The model under review builds one solid part; all positions refer to its coordinate system, in mm. A direction names the side the tool comes from. Coordinates: 2 decimals unless noted, no trailing zeros.
1) For line 1 (X direction, y = 10.75, z = -116); line 2 (Z direction, x = 81, y = 1); line 3 (Z direction, x = 41, y = 1), list the stretches that pass through material, from the lowest coordinate up.
2) For P1, Ø12.5, axis at x = -25.4, z = 50.8, coming from the +Y side; P2, Ø6, axis at x = -48.26, z = 31.75, coming from the -Y side; P3, Ø6, axis at x = 85, y = 6, coming from the +Z side, all flat-tipped, find the tip position at first contact; note any pin that passes through.
3) Machinability: for faces 5 (the cylindrical face through (0.151, 7.982, 105.794)), 6 (the cylindrical face through (-51.302, 3.187, 33.332)), 7 (the flat face through (124, 0, 30)), which of the approach directions +Z, -Z, +X, -X, +Y, -Y give a long, thin tool a straight path to every point of the face, cutting with its end or side? Answer none if there is none.
4) Mouldability with a two-part tool opening along Z and no side actions: class faces 1 (the cylindrical face through (60.55, 3.19, -0.45)), 2 (the cylindrical face through (136.38, 8.92, -30.28)), 3 (the flat face through (-2, 11.112, 2)), 4 (the cylindrical face through (-51.302, 3.187, -30.168)) as released by +Z, released by -Z, zero draft, split by the parting line, or undercut.
from build123d import *

# Parameters (mm, degrees)
SKETCH2_R          = 6.858
CUT_EXTRUDE1_DEPTH = 198.877910986
SKETCH3_R          = 25.4
SKETCH3_R_2        = 31.75
CUT_EXTRUDE3_DEPTH = 198.877910986
CUT_EXTRUDE4_START = -4.826
SKETCH4_R          = 3.429
CUT_EXTRUDE4_DEPTH = 6.35
SKETCH6_R          = 3.429
CUT_EXTRUDE6_DEPTH = 6.35


with BuildPart() as part:
    # Sketch1 → Revolve2 (revolve)
    with BuildSketch(Plane.XY, mode=Mode.PRIVATE) as revolve2_sk:
        with BuildLine():
            ThreePointArc((139.7, 6.7945), (136.8425, 3.937), (139.7, 1.0795))
            Line((139.7, 1.0795), (139.7, 0))
            Line((139.7, 0), (127, 0))
            Line((127, 0), (127, 2.54))
            Line((127, 2.54), (120.65, 2.54))
            Line((120.65, 2.54), (120.65, 0))
            Line((120.65, 0), (0, 0))
            Line((0, 0), (0, 11.1125))
            Line((0, 11.1125), (130.81, 11.1125))
            Line((130.81, 11.1125), (130.81, 9.8425))
            Line((130.81, 9.8425), (137.16, 9.8425))
            Line((137.16, 9.8425), (137.16, 11.1125))
            Line((137.16, 11.1125), (139.7, 11.1125))
            Line((139.7, 11.1125), (139.7, 6.7945))
        make_face()
    revolve(revolve2_sk.sketch.rotate(Axis((0, 28.20697446, 0), (0, -1, 0)), 90), axis=Axis((0, 28.20697446, 0), (0, -1, 0)))

    # Sketch2 → Cut-Extrude1 (cut, through all)
    with BuildSketch(Plane(origin=(0, 11.1125, 0), x_dir=(1, 0, 0), z_dir=(0, 1, 0))):
        with Locations(Location((-25.4, -50.8, 0), (0, 0, 270))):
            Circle(SKETCH2_R)
        with Locations(Location((25.4, -50.8, 0), (0, 0, 270))):
            Circle(SKETCH2_R)
    extrude(amount=-CUT_EXTRUDE1_DEPTH, mode=Mode.SUBTRACT)

    # Sketch3 → Cut-Extrude3 (cut, through all)
    with BuildSketch(Plane(origin=(0, 11.1125, 0), x_dir=(1, 0, 0), z_dir=(0, 1, 0))):
        with Locations(Location((0, 50.8, 0), (0, 0, 270))):
            Circle(SKETCH3_R)
        with Locations(Location((-82.55, 0, 0), (0, 0, 270))):
            Circle(SKETCH3_R_2)
    extrude(amount=-CUT_EXTRUDE3_DEPTH, mode=Mode.SUBTRACT)

    # Sketch4 → Cut-Extrude4 (cut)
    with BuildSketch(Plane(origin=(0, 11.1125, 0), x_dir=(1, 0, 0), z_dir=(0, 1, 0)).offset(CUT_EXTRUDE4_START)):
        with Locations(Location((57.15, 0, 0), (0, 0, 270))):
            Circle(SKETCH4_R)
        with Locations(Location((-48.26, -31.75, 0), (0, 0, 270))):
            Circle(SKETCH4_R)
        with Locations(Location((-48.26, 31.75, 0), (0, 0, 270))):
            Circle(SKETCH4_R)
    extrude(amount=-CUT_EXTRUDE4_DEPTH, mode=Mode.SUBTRACT)

    # Sketch6 → Cut-Extrude6 (cut)
    with BuildSketch(Plane(origin=(0, 11.1125, 0), x_dir=(1, 0, 0), z_dir=(0, 1, 0))):
        with Locations(Location((0, -109.22, 0), (0, 0, 270))):
            Circle(SKETCH6_R)
        with Locations(Location((82.55, 76.127347805, 0), (0, 0, 270))):
            Circle(SKETCH6_R)
        with Locations(Location((-82.55, 76.127347805, 0), (0, 0, 270))):
            Circle(SKETCH6_R)
    extrude(amount=-CUT_EXTRUDE6_DEPTH, mode=Mode.SUBTRACT)


solid = part.part
Geometry results:
1. line 1: x = -77.85 to -73.19, -60.46 to 60.46, 73.19 to 77.85
1. line 2: z = -113.82 to -97.82, -89.42 to 89.42, 97.82 to 113.82
1. line 3: z = -133.55 to -120.2, -113.47 to 113.47, 120.2 to 133.55
2. P1: passes through
2. P2: stops at y = 6.29
2. P3: stops at z = 113.02
3. face 5: +Y
3. face 6: -Y
3. face 7: +Z, -Z, +X, -X, -Y
4. face 1: undercut
4. face 2: split by the parting line
4. face 3: zero draft
4. face 4: undercut
